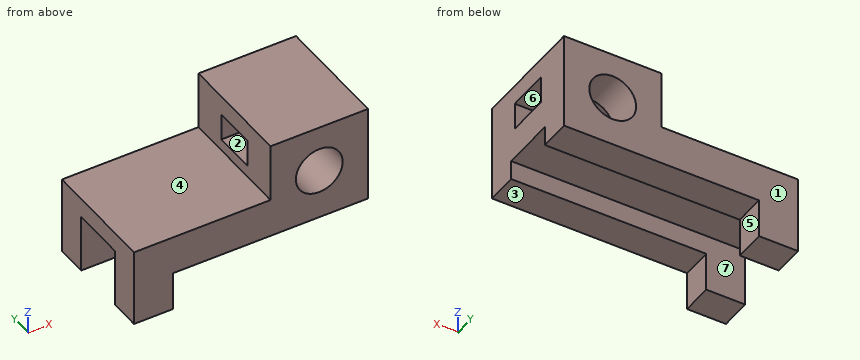
```python
from build123d import *

# Parameters (mm, degrees)
F0_R     = 120
F1_DEPTH = 600
F2_W     = 220
F2_H     = 140
F3_DEPTH = 1200.001
F4_W     = 280
F4_H     = 300
F5_DEPTH = 1200.001


with BuildPart() as f1:
    # F0 (on Front) → F1 (new body)
    with BuildSketch(Plane.XZ):
        with Locations((350, 110)):
            Circle(F0_R)
        Polygon((600, 110), (600, 350), (100, 350), (100, 50), (-600, 50), (-600, -350), (-400, -350), (-400, -150), (600, -150), (600, 50), align=None)
        with Locations((350, 110)):
            Circle(F0_R, mode=Mode.SUBTRACT)
    extrude(amount=F1_DEPTH)

    # F2 (on face) → F3 (cut, through all)
    with BuildSketch(Plane.YZ.offset(600)):
        with Locations((-300, 180)):
            Rectangle(F2_W, F2_H)
    extrude(amount=-F3_DEPTH, mode=Mode.SUBTRACT)

    # F4 (on face) → F5 (cut, through all)
    with BuildSketch(Plane(origin=(-600, 0, 0), x_dir=(0, -1, 0), z_dir=(-1, 0, 0))):
        with Locations((300, -200)):
            Rectangle(F4_W, F4_H)
    extrude(amount=-F5_DEPTH, mode=Mode.SUBTRACT)


solid = f1.part
```
Here's how the part is built. I have some questions about the finished solid (model axes, mm). Face numbers are marked on the shaded views. A direction names the side the tool comes from. Coordinates: 2 decimals unless noted, no trailing zeros. Write each loop counter-clockwise with the first axis right and the second up, starting at its lowest first coordinate (ties: lowest second). Pieces come first, ordered by that corner, then holes. Notation, with made-up numbers: (40, -30.75) - (53, -30.75) arc R30 cw to (53, 6.25) - close; hole circle Ø8 at (-31, 73). An arc over 180 degrees is marked (long way). One line per item, written item: value.
1) Suppose I cut it at B-B on z = -228.5. Write out the boundary of the cut face in (x, y).
Model answer:
outline: (-600, -600) - (-400, -600) - (-400, -440) - (-600, -440) - close; (-600, -160) - (-400, -160) - (-400, 0) - (-600, 0) - close
2) I'm going to push flat-ended pins straight in: P1, Ø8, axis at x = -130.5, y = -402, coming from the +Z side; P2, Ø6, axis at y = -490, z = 181, coming from the -X side; P3, Ø12, axis at x = 276, y = -347, coming from the -Z side. Where does each tip first touch, or does it pass through?
Model answer:
P1: stops at z = 50
P2: stops at x = 100
P3: stops at z = -50
3) Suppose I cut it at A-A on x = 350. Write out the boundary of the cut face in (y, z).
Model answer:
outline: (-600, -150) - (-440, -150) - (-440, -50) - (-160, -50) - (-160, -150) - (0, -150) - (0, -10) - (-600, -10) - close; (-600, 230) - (-410, 230) - (-410, 250) - (-190, 250) - (-190, 230) - (0, 230) - (0, 350) - (-600, 350) - close
4) We'd pull the mould along Z, two halves only. Please class the marked faces 1, 2, 3 and 4: pulls with the +Z half, pulls with the -Z half, needs draft (parallel to the pull), parting line crosses it, or undercut.
Model answer:
face 1: needs draft
face 2: undercut
face 3: pulls with the -Z half
face 4: pulls with the +Z half
5) On a 3-axis mill with a long thin cutter (end or side, diameter ignored), from which of +Z, -Z, +X, -X, +Y, -Y can I reach the whole of each face in a straight line? I mean the marked faces 5, 6 and 7. Say none if no direction works.
Model answer:
face 5: -Z, +X, +Y, -Y
face 6: +X, -X
face 7: -Z, +X, -X
6) Suppose I cut it at D-D on x = -53.5. Write out the boundary of the cut face in (y, z).
Model answer:
outline: (-600, -150) - (-440, -150) - (-440, -50) - (-160, -50) - (-160, -150) - (0, -150) - (0, 50) - (-600, 50) - close
7) Suppose I cut it at C-C on y = -489. Write out the boundary of the cut face in (x, z).
Model answer:
outline: (-600, -350) - (-400, -350) - (-400, -150) - (600, -150) - (600, 350) - (100, 350) - (100, 50) - (-600, 50) - close; hole circle Ø240 at (350, 110)
8) I need wall thicknesses on line 1 along Z through (x, y) = (350, -334); line 2 along Y through (x, z) = (38, -112); line 3 along Z through (x, y) = (544, -219). Which ranges of each line are inside material? Lowest first, please.
Model answer:
line 1: z = -50 to -10, 250 to 350
line 2: y = -600 to -440, -160 to 0
line 3: z = -50 to 110, 250 to 350
